from build123d import *

# Parameters (mm, degrees)
SKETCH1_W           = 18
SKETCH1_H           = 5
BOSS_EXTRUDE1_DEPTH = 1.5
SKETCH2_W           = 18
SKETCH2_H           = 2.5
SKETCH2_W_2         = 4.8
SKETCH2_H_2         = 1
BOSS_EXTRUDE3_DEPTH = 4
SKETCH4_W           = 18
SKETCH4_H           = 2.5
BOSS_EXTRUDE4_DEPTH = 4.5
SKETCH6_W           = 5
SKETCH6_H           = 10
BOSS_EXTRUDE5_DEPTH = 1.5
SKETCH7_W           = 5
SKETCH7_H           = 10
BOSS_EXTRUDE6_DEPTH = 1.5


with BuildPart() as part:
    # Sketch1 → Boss-Extrude1 (new body)
    with BuildSketch(Plane(origin=(0, 0, 0), x_dir=(1, 0, 0), z_dir=(0, 1, 0))):
        with Locations((3.151785714, 0.111607143)):
            Rectangle(SKETCH1_W, SKETCH1_H)
    extrude(amount=BOSS_EXTRUDE1_DEPTH)

    # Sketch2 → Boss-Extrude3 (add)
    with BuildSketch(Plane(origin=(0, 1.5, 0), x_dir=(1, 0, 0), z_dir=(0, 1, 0))):
        with Locations((3.151785714, -1.138392857)):
            Rectangle(SKETCH2_W, SKETCH2_H)
        with Locations((-3.448214286, 2.111607143)):
            Rectangle(SKETCH2_W_2, SKETCH2_H_2)
        with Locations((9.751785714, 2.111607143)):
            Rectangle(SKETCH2_W_2, SKETCH2_H_2)
    extrude(amount=BOSS_EXTRUDE3_DEPTH)

    # Sketch4 → Boss-Extrude4 (add)
    with BuildSketch(Plane(origin=(0, 5.5, 0), x_dir=(1, 0, 0), z_dir=(0, 1, 0))):
        with Locations((3.151785714, -1.138392857)):
            Rectangle(SKETCH4_W, SKETCH4_H)
    extrude(amount=BOSS_EXTRUDE4_DEPTH)

    # Sketch6 → Boss-Extrude5 (add)
    with BuildSketch(Plane(origin=(12.151785714, 0, 0), x_dir=(0, 0, -1), z_dir=(1, 0, 0))):
        with Locations((0.111607143, 5)):
            Rectangle(SKETCH6_W, SKETCH6_H)
    extrude(amount=BOSS_EXTRUDE5_DEPTH)

    # Sketch7 → Boss-Extrude6 (add)
    with BuildSketch(Plane.ZY.offset(5.848214286)):
        with Locations((-0.111607143, 5)):
            Rectangle(SKETCH7_W, SKETCH7_H)
    extrude(amount=BOSS_EXTRUDE6_DEPTH)


solid = part.part
Could you check a few things on this model? Use its own coordinates, in mm. A direction names the side the tool comes from. Coordinates: 2 decimals unless noted, no trailing zeros. Order: outer loops, then holes, each group sorted by start corner. A loop starts at its lowest first (then second) coordinate and runs counter-clockwise, first axis right, second up. Notation, with made-up numbers: (-11, -10) -> (46, -10) arc R8 ccw to (46, -4) -> close; hole circle Ø2 at (89.25, 34.5). An arc over 180 degrees is marked (long way). One line per item, written item: value. Start each with the question number.
1) Imagine slicing it at B-B on x = 8.25. List the corners of the cut face in (y, z) for me, plus the area to 4 significant figures.
2) Imagine slicing it at A-A on z = -2.1. List the corners of the cut face in (x, y) for me.
3) Imagine slicing it at C-C on y = 8.75. List the corners of the cut face in (x, z) for me, plus the area to 3 significant figures.
4) Imagine slicing it at D-D on x = 1. List the corners of the cut face in (y, z) for me.
5) If I drill on L1, parallel to Z at x = -4.5, y = 3; L2, parallel to X at y = 8.75, z = -1.25; L3, parallel to Z at x = -0.25, y = 5, over which ranges is the centre line in solid material (lowest first)? Write a range as [from, to].
6) We'd pull the mould along Z, two halves only. Please class faces 1 (the flat face through (3.3, 0.5, -2.612)), 2 (the flat face through (10, 3, -1.612)), 3 (the flat face through (3, 5, 2.388)), 4 (the flat face through (13.652, 5, 0)): +Z half, -Z half, draft (parallel to the pull), parting line (faces both ways), or undercut.
7) Which directions (+Z, -Z, +X, -X, +Y, -Y) give clear straight access to the entire face, cutting with the end or side of a thin tool? Please do faces 5 (the flat face through (-3, 3, -1.612)), 6 (the flat face through (3, 10, 1)), 7 (the flat face through (-3, 5.5, -2)).
8) I'm going to push flat-ended pins straight in: pin 1 (1.1 mm diameter, centred on x = -2.5, z = -2, fed in from +Y); pin 2 (3 mm diameter, centred on x = -4, y = 8.5, fed in from -Z). Where does each tip first touch, or does it pass through?
Answer list:
1. outline: (0, -2.61) -> (5.5, -2.61) -> (5.5, -1.61) -> (1.5, -1.61) -> (1.5, -0.11) -> (10, -0.11) -> (10, 2.39) -> (0, 2.39) -> close
1. area: 32.75 mm2
2. outline: (-7.35, 0) -> (13.65, 0) -> (13.65, 10) -> (12.15, 10) -> (12.15, 5.5) -> (7.35, 5.5) -> (7.35, 1.5) -> (-1.05, 1.5) -> (-1.05, 5.5) -> (-5.85, 5.5) -> (-5.85, 10) -> (-7.35, 10) -> close
3. outline: (-7.35, -2.61) -> (-5.85, -2.61) -> (-5.85, -0.11) -> (12.15, -0.11) -> (12.15, -2.61) -> (13.65, -2.61) -> (13.65, 2.39) -> (-7.35, 2.39) -> close
3. area: 60.0 mm2
4. outline: (0, -2.61) -> (1.5, -2.61) -> (1.5, -0.11) -> (10, -0.11) -> (10, 2.39) -> (0, 2.39) -> close
5. L1: z = [-2.61, -1.61], [-0.11, 2.39]
5. L2: x = [-7.35, -5.85], [12.15, 13.65]
5. L3: z = [-0.11, 2.39]
6. face 1: -Z half
6. face 2: undercut
6. face 3: +Z half
6. face 4: draft
7. face 5: +Y
7. face 6: +Z, -Z, +X, -X, +Y
7. face 7: -Z, +Y
8. pin 1: stops at y = 5.5
8. pin 2: stops at z = -0.11
